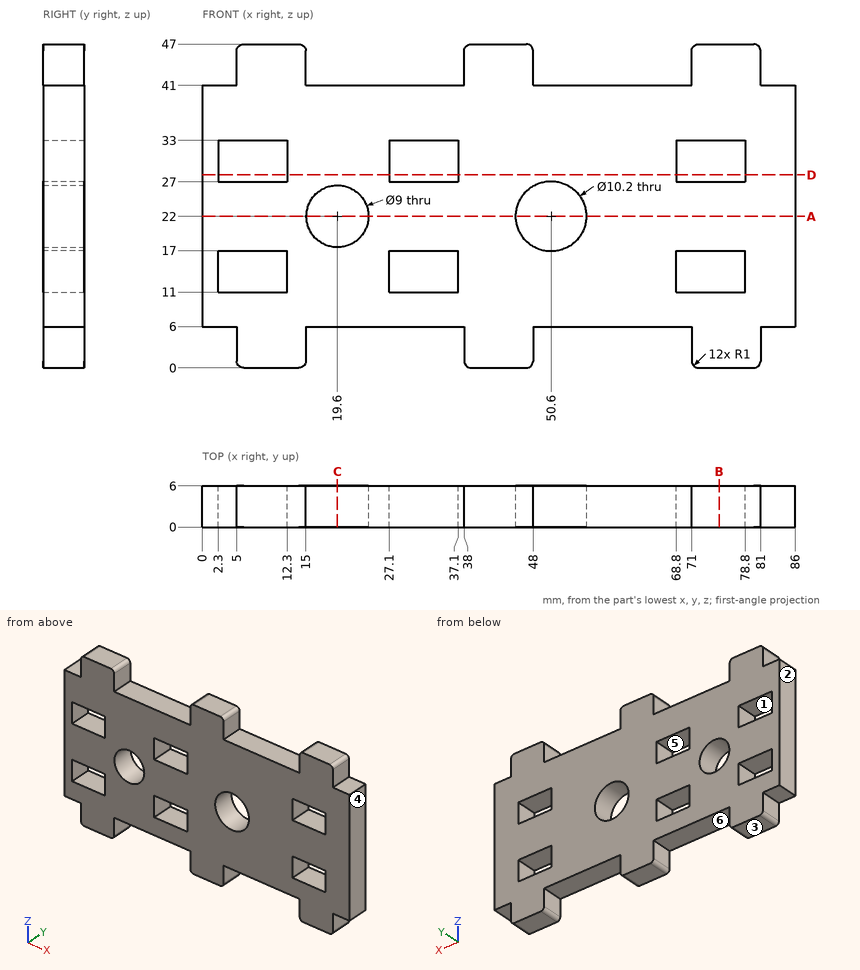
Could you check a few things on this drawing? It's one solid part, dimensions in mm from its lowest x, y, z. A direction names the side the tool comes from. Coordinates: 2 decimals unless noted, no trailing zeros. Order: outer loops, then holes, each group sorted by start corner. A loop starts at its lowest first (then second) coordinate and runs counter-clockwise, first axis right, second up.
1) We'd pull the mould along X, two halves only. Please class the marked faces 1, 2 and 3: +X half, -X half, draft (parallel to the pull), parting line (faces both ways), or undercut.
2) Imagine slicing it at C-C on x = 19.6. List the corners of the cut face in (y, z) for me.
3) Imagine slicing it at A-A on z = 22. List the corners of the cut face in (x, y) for me.
4) I need wall thicknesses on line 1 (X direction, y = 3.45, z = 30); line 2 (X direction, y = 0.95, z = 5.5); line 3 (X direction, y = 2.9, z = 22). Which ranges of each line are inside material? Lowest first, please.
5) Will these pins go through, and if not, where does the flat tip stop? pin 1 (2.5 mm diameter, centred on y = 3, z = 43, fed in from -X); pin 2 (1.5 mm diameter, centred on y = 4.5, z = 4.5, fed in from +X); pin 3 (3 mm diameter, centred on x = 24, y = 4, fed in from -Z).
6) Imagine slicing it at D-D on z = 28. List the corners of the cut face in (x, y) for me, and give its area (3 significant figures).
7) Imagine slicing it at B-B on x = 75. List the corners of the cut face in (y, z) for me, and give its area (3 significant figures).
8) Which directions (+Z, -Z, +X, -X, +Y, -Y) give clear straight access to the entire face, cutting with the end or side of a thin tool? Please do the marked faces 4, 5 and 6.
Response values:
1. face 1: undercut
1. face 2: -X half
1. face 3: draft
2. outline: (0, 6) - (6, 6) - (6, 17.5) - (0, 17.5) - close; (0, 26.5) - (6, 26.5) - (6, 41) - (0, 41) - close
3. outline: (0, 0) - (15.1, 0) - (15.1, 6) - (0, 6) - close; (24.1, 0) - (45.5, 0) - (45.5, 6) - (24.1, 6) - close; (55.7, 0) - (86, 0) - (86, 6) - (55.7, 6) - close
4. line 1: x = 0 to 2.3, 12.3 to 27.1, 37.1 to 68.8, 78.8 to 86
4. line 2: x = 5 to 15, 38 to 48, 71 to 81
4. line 3: x = 0 to 15.1, 24.1 to 45.5, 55.7 to 86
5. pin 1: stops at x = 5
5. pin 2: stops at x = 81
5. pin 3: stops at z = 6
6. outline: (0, 0) - (2.3, 0) - (2.3, 6) - (0, 6) - close; (12.3, 0) - (27.1, 0) - (27.1, 6) - (12.3, 6) - close; (37.1, 0) - (68.8, 0) - (68.8, 6) - (37.1, 6) - close; (78.8, 0) - (86, 0) - (86, 6) - (78.8, 6) - close
6. area: 336 mm2
7. outline: (0, 0) - (6, 0) - (6, 11) - (0, 11) - close; (0, 17) - (6, 17) - (6, 27) - (0, 27) - close; (0, 33) - (6, 33) - (6, 47) - (0, 47) - close
7. area: 210 mm2
8. face 4: +Z, -Z, +X, +Y, -Y
8. face 5: +Y, -Y
8. face 6: -Z, +Y, -Y
